from build123d import *

# Parameters (mm, degrees)
F0_W      = 128.3
F0_H      = 66.85852
F0_W_2    = 116.3
F0_H_2    = 54.85852
F1_DEPTH  = 70
F2_DEPTH  = 2
F4_DEPTH  = 130
F5_W      = 9
F5_H      = 12.5
F6_DEPTH  = 7
F5_W_2    = 15
F5_H_2    = 6.5
F7_DEPTH  = 7
F9_DEPTH  = 5
F11_DEPTH = 5
F12_W     = 23.2212013245
F12_H     = 1.5
F13_DEPTH = 17.5
F15_R     = 1.35
F16_DEPTH = 9.5
F18_DEPTH = 141.4
F19_DEPTH = 133.9
F21_DEPTH = 128.26
F22_DEPTH = 9
F23_R     = 2.75
F24_DEPTH = 25


with BuildPart() as f1:
    # F0 (on Top) → F1 (new body)
    with BuildSketch(Plane.XY):
        Rectangle(F0_W, F0_H)
        Rectangle(F0_W_2, F0_H_2, mode=Mode.SUBTRACT)
    extrude(amount=F1_DEPTH)

    # F0 (on Top) → F2 (join)
    with BuildSketch(Plane.XY):
        Rectangle(F0_W_2, F0_H_2)
    extrude(amount=F2_DEPTH)

    # F3 (on face) → F4 (cut)
    with BuildSketch(Plane.YZ.offset(64.15)):
        Polygon((-33.42926, 14.4301047549), (33.42926, 70), (-33.42926, 70), align=None)
    extrude(amount=-F4_DEPTH, mode=Mode.SUBTRACT)

    # F5 (on face) → F6 (cut)
    with BuildSketch(Plane.YZ.offset(64.15)):
        with Locations((20.92926, 13.25)):
            Rectangle(F5_W, F5_H)
    extrude(amount=-F6_DEPTH, mode=Mode.SUBTRACT)

    # F5 (on face) → F7 (cut)
    with BuildSketch(Plane.YZ.offset(64.15)):
        with Locations((0.0932381302, 5.25)):
            Rectangle(F5_W_2, F5_H_2)
    extrude(amount=-F7_DEPTH, mode=Mode.SUBTRACT)

    # F8 (on face) → F9 (cut)
    with BuildSketch(Plane(origin=(58.15, 0, 0), x_dir=(0, -1, 0), z_dir=(-1, 0, 0))):
        Polygon((-8.8432381302, 13.5), (-8.8432381302, 2), (-7.5932381302, 2), (-7.5932381302, 8.5), (7.4067618698, 8.5), (7.4067618698, 2), (8.6567618698, 2), (8.6567618698, 13.5), align=None)
    extrude(amount=-F9_DEPTH, mode=Mode.SUBTRACT)

    # F10 (on face) → F11 (join)
    with BuildSketch(Plane.XY.offset(2)):
        Polygon((33.15, 9.5932381302), (33.15, 7.5932381302), (33.15, -7.4067618698), (33.15, -9.4067618698), (43.15, -9.4067618698), (43.15, -7.4067618698), (35.15, -7.4067618698), (35.15, 7.5932381302), (43.15, 7.5932381302), (43.15, 9.5932381302), align=None)
    extrude(amount=F11_DEPTH)

    # F12 (on face) → F13 (join)
    with BuildSketch(Plane.XY.offset(2)):
        with Locations((-46.5393993378, 7.67926)):
            Rectangle(F12_W, F12_H)
        Polygon((9.35, 27.42926), (7.85, 27.42926), (7.85, 8.42926), (-2.2495171815, 8.42926), (-2.2495171815, 6.92926), (9.35, 6.92926), (9.35, 8.42926), align=None)
    extrude(amount=F13_DEPTH)

    # F15 (on offset) → F16 (cut)
    with BuildSketch(Plane(origin=(0, -21.2629991115, 25.582424532), x_dir=(1, 0, 0), z_dir=(0, -0.6391959003, 0.7690439526))):
        with Locations((-61.15, -13.4849064425)):
            Circle(F15_R)
        with Locations((61.15, -13.4849064425)):
            Circle(F15_R)
    extrude(amount=-F16_DEPTH, mode=Mode.SUBTRACT)

    # F17 (on face) → F18 (cut)
    with BuildSketch(Plane.YZ.offset(64.15)):
        Polygon((92.054369559, 57.1661034537), (92.054369559, 115.2663065398), (-2.9636703822, 115.2663065398), (-2.9636703822, 57.1661034537), (17.9882496267, 57.1661034537), (33.42926, 70), (33.42926, 57.1661034537), align=None)
    extrude(amount=-F18_DEPTH, mode=Mode.SUBTRACT)

    # F17 (on face) → F19 (cut)
    with BuildSketch(Plane.YZ.offset(64.15)):
        Polygon((17.9882496267, 57.1661034537), (33.42926, 57.1661034537), (33.42926, 70), align=None)
    extrude(amount=-F19_DEPTH, mode=Mode.SUBTRACT)

    # F20 (on face) → F21 (join)
    with BuildSketch(Plane.YZ.offset(64.15)):
        Polygon((17.9882496267, 57.1661034537), (13.2818869306, 53.254379383), (33.42926, 43.7797382474), (33.42926, 57.1661034537), align=None)
    extrude(amount=-F21_DEPTH)

    # F15 (on offset) → F22 (cut)
    with BuildSketch(Plane(origin=(0, -21.2629991115, 25.582424532), x_dir=(1, 0, 0), z_dir=(0, -0.6391959003, 0.7690439526))):
        with Locations((61.15, 47.3736135575)):
            Circle(F15_R)
        with Locations((-61.15, 47.3736135575)):
            Circle(F15_R)
    extrude(amount=-F22_DEPTH, mode=Mode.SUBTRACT)

    # F23 (on face) → F24 (cut)
    with BuildSketch(Plane.XZ.offset(-27.42926)):
        with Locations((23.2078029529, 6.984276909)):
            Circle(F23_R)
        with Locations((31.4362019996, 6.984276909)):
            Circle(F23_R)
    extrude(amount=-F24_DEPTH, mode=Mode.SUBTRACT)


solid = f1.part
Read the model definition and answer for the solid it produces. Units are mm, in the model's axes. A direction names the side the tool comes from. Give positions to 0.01 mm unless a question says otherwise; leave off trailing zeros. Write each loop counter-clockwise with the first axis right and the second up, starting at its lowest first coordinate (ties: lowest second). Pieces come first, ordered by that corner, then holes. Notation, with made-up numbers: M 88,40 L 113,40 A30 ccw 113,69 Z; hole C -20,23 d8. An arc over 180 degrees is marked long. One line per item, written item: value. Start each with the question number.
(1) Find section B-B (x = -8.5). Determine the outline of the cut face in (y, z), plus the area to 3 significant figures.
(2) Flat-ended cylindrical pins translate along their axes: pin 1 Ø2 at (x, z) = (31.5, 18) entering from -Y; pin 2 Ø22.5 at (x, z) = (14.5, 29) entering from -Y; pin 3 Ø11 at (x, y) = (36, 0) entering from +Z. Find the tip coordinate at first contact, or state that the pin passes through.
(3) Find section D-D (x = 23). Determine the outline of the cut face in (y, z), plus the area to 3 significant figures.
(4) Find the intervals of material crossed by line 1 (X direction, y = 12, z = 13); line 2 (Y direction, x = -2, z = 4); line 3 (X direction, y = 10.5, z = 28.5), in increasing order.
(5) Determine the mould class of faces 1 (the cylindrical face through (33.977, 30.387, 5.931)), 2 (the flat face through (-1, 33.429, 28)), 3 (the flat face through (35.15, 0, 4)) for opening direction Y: pulls with the +Y half, pulls with the -Y half, needs draft (parallel to the pull), parting line crosses it, or undercut.
(6) Find section A-A (y = 1.5). Determine the outline of the cut face in (x, z), plus the area to 3 significant figures.
(7) A tool of negligible diameter and unlimited length cuts with its end or side. For faces 4 (the flat face through (-47, 6.929, 11)), 5 (the flat face through (61, 25.429, 13)), 6 (the flat face through (-58.15, 6, 22)), 7 (the flat face through (8, 13, 19.5)), from which of +Z, -Z, +X, -X, +Y, -Y can it reach the whole face along a straight path? Write none if from no direction.
(8) Find section C-C (y = 11.5). Determine the outline of the cut face in (x, z), plus the area to 3 significant figures.
Results below:
1. outline: M -33.43,0 L 33.43,0 L 33.43,57.17 L 17.99,57.17 L 13.28,53.25 L 27.43,46.6 L 27.43,2 L -27.43,2 L -27.43,19.42 L -33.43,14.43 Z
1. area: 647 mm^2
2. pin 1: stops at y = -30.34
2. pin 2: stops at y = -29.43
2. pin 3: stops at z = 7
3. outline: M -33.43,0 L 33.43,0 L 33.43,4.24 L 27.43,4.24 L 27.43,2 L -27.43,2 L -27.43,19.42 L -33.43,14.43 Z; M 13.28,53.25 L 27.43,46.6 L 27.43,9.73 L 33.43,9.73 L 33.43,57.17 L 17.99,57.17 Z
3. area: 615 mm^2
4. line 1: x = -64.15 to -58.15, 7.85 to 9.35, 58.15 to 64.15
4. line 2: y = -33.43 to -27.43, 6.93 to 8.43, 27.43 to 33.43
4. line 3: x = -64.15 to -58.15, 58.15 to 64.15
5. face 1: needs draft
5. face 2: pulls with the +Y half
5. face 3: undercut
6. outline: M -64.15,0 L 64.15,0 L 64.15,2 L 35.15,2 L 35.15,7 L 33.15,7 L 33.15,2 L -58.15,2 L -58.15,43.46 L -64.15,43.46 Z; M 58.15,13.5 L 63.15,13.5 L 63.15,8.5 L 64.15,8.5 L 64.15,43.46 L 58.15,43.46 Z
6. area: 700 mm^2
7. face 4: +Z
7. face 5: +X
7. face 6: none
7. face 7: -Y
8. outline: M -64.15,0 L 64.15,0 L 64.15,51.77 L 58.15,51.77 L 58.15,2 L 9.35,2 L 9.35,19.5 L 7.85,19.5 L 7.85,2 L -58.15,2 L -58.15,51.77 L -64.15,51.77 Z
8. area: 880 mm^2
